from build123d import *

# Parameters (mm, degrees)
SKETCH1_W           = 6.73955421
SKETCH1_H           = 6.812677774
SKETCH1_R           = 2.51
BOSS_EXTRUDE1_DEPTH = 30.13


with BuildPart() as part:
    # Sketch1 → Boss-Extrude1 (new body)
    with BuildSketch(Plane.XY):
        Rectangle(SKETCH1_W, SKETCH1_H)
        Circle(SKETCH1_R, mode=Mode.SUBTRACT)
        with BuildLine():
            add(Edge.make_bspline(
                [(28.500199806, -7.5), (3.369777105, -3.406338887)],
                knots=[0, 0, 1, 1], degree=1))
            Line((3.369777105, -3.406338887), (3.369777105, 3.406338887))
            add(Edge.make_bspline(
                [(28.143383308, -4.373850119), (16.666117653, 2.316528631), (3.369777105, 3.406338887)],
                knots=[0, 0, 0, 1, 1, 1], degree=2))
            Line((28.143383308, -4.373850119), (33.109649153, -6.51665119))
            Line((33.109649153, -6.51665119), (33.500199806, -7.5))
            Line((33.500199806, -7.5), (28.500199806, -7.5))
        make_face()
    extrude(amount=BOSS_EXTRUDE1_DEPTH)


solid = part.part
Design review of the part built by this model. Coordinates are the model's own, in mm. A direction names the side the tool comes from. Round coordinates to 2 decimals unless told otherwise and drop trailing zeros. Write each loop counter-clockwise with the first axis right and the second up, starting at its lowest first coordinate (ties: lowest second). Pieces come first, ordered by that corner, then holes. Notation, with made-up numbers: M 15,69.5 L 37,69.5 A13 ccw 37,89.5 Z; hole C 60.5,7 d11. An arc over 180 degrees is marked long. One line per item, written item: value. Start each with the question number.
1. Take a section at A-A on x = 0. State the section outline as (y, z) points.
2. Draft analysis for pull direction Y (two halves, no side actions). For faces 1 (the face through (-0.54, -2.45, 14.85)), 2 (the face through (11, -2, 30.13)), 3 (the face through (33.3, -7, 14.9)), state which applies: pulls with the +Y half, pulls with the -Y half, needs draft (parallel to the pull), parting line crosses it, or undercut.
3. For faces 4 (the face through (0, 3.406, 15)), 5 (the face through (0, -3.406, 15)), list the 3-axis set-ups (+Z, -Z, +X, -X, +Y, -Y) from which the entire face can be reached by the end or side of a thin tool; tool diameter is ignored.
4. Clearance check with flat-ended pins moving along their axes: P1, Ø5, axis at y = -3, z = 5.5, coming from the +X side; P2, Ø3.5, axis at x = 0.5, z = 8.5, coming from the -Y side; P3, Ø5, axis at x = 25, z = 9.5, coming from the +Y side. State where each tip first meets the part, or that it passes through.
5. To check wall thickness, follow probe 1 along Y at (x, z) = (0, 15); probe 2 along X at (y, z) = (-1, 26); probe 3 along X at (y, z) = (-2, 10.5). State the ranges of each line that lie inside material, in increasing order. Write a range as from..to.
Computed:
1. outline: M -3.41,0 L -2.51,0 L -2.51,30.13 L -3.41,30.13 Z; M 2.51,0 L 3.41,0 L 3.41,30.13 L 2.51,30.13 Z
2. face 1: undercut
2. face 2: needs draft
2. face 3: pulls with the +Y half
3. face 4: +Z, -Z, +X, -X, +Y
3. face 5: +Z, -Z, -X, -Y
4. P1: stops at x = 30.75
4. P2: stops at y = -3.41
4. P3: stops at y = -1.47
5. probe 1: y = -3.41..-2.51, 2.51..3.41
5. probe 2: x = -3.37..-2.3, 2.3..21.42
5. probe 3: x = -3.37..-1.52, 1.52..23.65
